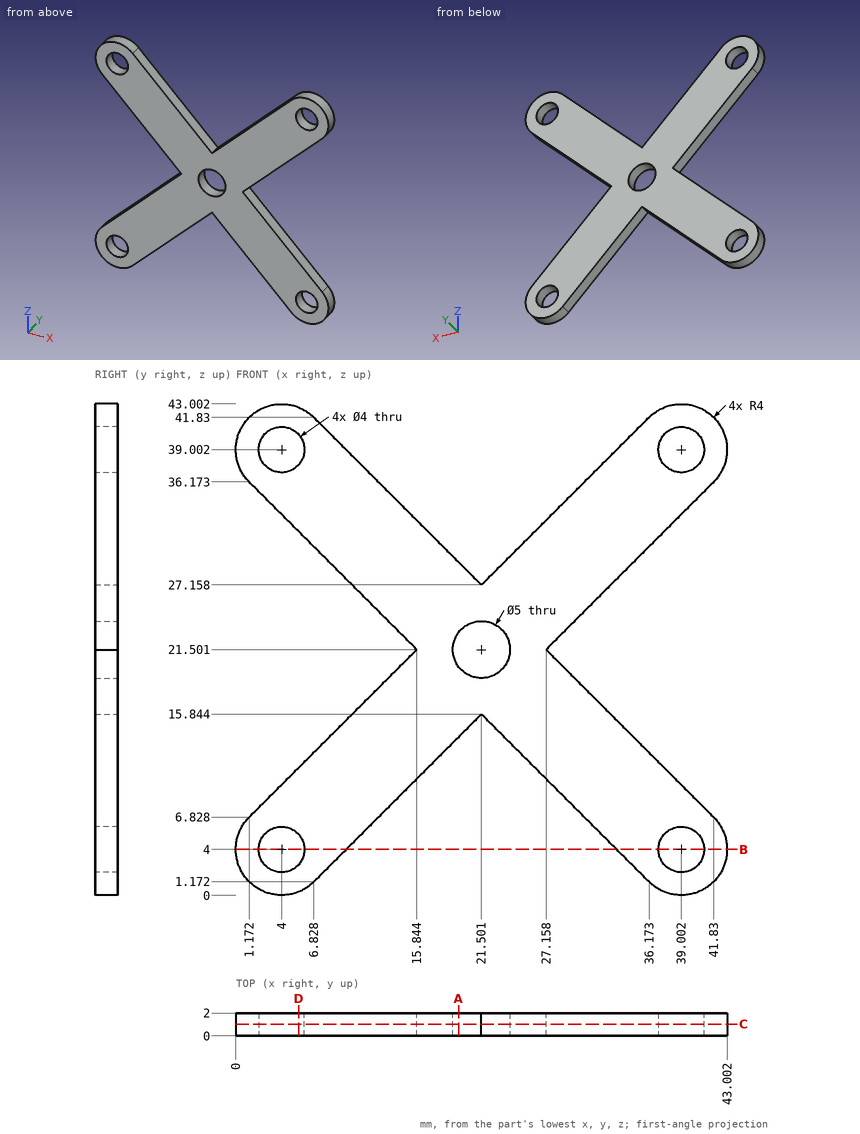
Input: dimensioned drawing with shaded views. Units: mm. Origin: part minimum x, y, z. Give positions to 0.01 mm unless a question says otherwise; leave off trailing zeros. Loops run counter-clockwise (first coordinate to the right, second up) from the corner with the lowest first, then second, coordinate; pieces in that order, holes last. Notation, with made-up numbers: (33, -8) - (90, -8) arc R21 ccw to (90, 14) - close; hole circle Ø4 at (-16, 47). An arc over 180 degrees is marked (long way). Answer as CSV lines item,"result". Start each with the question number.
(1) Section query A-A (x = 19.5). Output: boundary loops of the cut face in (y, z).
(2) Section query B-B (z = 4). Output: boundary loops of the cut face in (x, y) (1 decimal).
(3) Ray query, line 1 along Z through (x, y) = (4, 0.95) (1 decimal); line 2 along X through (y, z) = (0.9, 5.5) (1 decimal); line 3 along Z through (x, y) = (30, 0.4) (1 decimal). Return the intervals inside material, ascending. Write a range as [from, to].
(4) Section query D-D (x = 5.5). Output: boundary loops of the cut face in (y, z) (1 decimal).
(5) Section query C-C (y = 1.05). Output: boundary loops of the cut face in (x, z).
(6) Pin query (flat end, axial travel): P1, Ø3.5, axis at x = 4, z = 39, coming from the +Y side; P2, Ø1, axis at y = 1, z = 11.5, coming from the +X side. Return the tip coordinate at first contact, or that it passes through.
Worked answers:
1,outline,"(0, 13.84) - (2, 13.84) - (2, 20) - (0, 20) - close; (0, 23) - (2, 23) - (2, 29.16) - (0, 29.16) - close"
2,outline,"(0, 0) - (2, 0) - (2, 2) - (0, 2) - close; (6, 0) - (9.7, 0) - (9.7, 2) - (6, 2) - close; (33.3, 0) - (37, 0) - (37, 2) - (33.3, 2) - close; (41, 0) - (43, 0) - (43, 2) - (41, 2) - close"
3,line 1,"z = [0, 2], [6, 9.7], [33.3, 37], [41, 43]"
3,line 2,"x = [0.3, 2.7], [5.3, 11.2], [31.8, 37.7], [40.3, 42.7]"
3,line 3,"z = [7.3, 18.7], [24.3, 35.7]"
4,outline,"(0, 0.3) - (2, 0.3) - (2, 2.7) - (0, 2.7) - close; (0, 5.3) - (2, 5.3) - (2, 11.2) - (0, 11.2) - close; (0, 31.8) - (2, 31.8) - (2, 37.7) - (0, 37.7) - close; (0, 40.3) - (2, 40.3) - (2, 42.7) - (0, 42.7) - close"
5,outline,"(1.17, 6.83) arc R4 ccw to (6.83, 1.17) - (21.5, 15.84) - (36.17, 1.17) arc R4 ccw to (41.83, 6.83) - (27.16, 21.5) - (41.83, 36.17) arc R4 ccw to (36.17, 41.83) - (21.5, 27.16) - (6.83, 41.83) arc R4 ccw to (1.17, 36.17) - (15.84, 21.5) - close; hole circle Ø4 at (4, 4); hole circle Ø4 at (4, 39); hole circle Ø5 at (21.5, 21.5); hole circle Ø4 at (39, 4); hole circle Ø4 at (39, 39)"
6,P1,"passes through"
6,P2,"stops at x = 37.66"
